For this review, take the finished solid that the model builds, in its own axes (mm). A direction names the side the tool comes from. Round coordinates to 2 decimals unless told otherwise and drop trailing zeros. Write each loop counter-clockwise with the first axis right and the second up, starting at its lowest first coordinate (ties: lowest second). Pieces come first, ordered by that corner, then holes.
from build123d import *

# Parameters (mm, degrees)
F0_R            = 10
F1_DEPTH        = 4
F3_DEPTH        = 4.001
F3_COPIES_COUNT = 9


# Not quite as in the source:
# - a pattern or mirror of a feature is missing from the dataset's text; its kind, count and spacing are read off the source's solid


with BuildPart() as f1:
    # F0 (on Top) → F1 (new body)
    with BuildSketch(Plane.XY):
        Circle(F0_R)
    extrude(amount=F1_DEPTH)

    # F2 (on face) → F3 (cut, through all)
    with BuildSketch(Plane.XY.offset(4)):
        with BuildLine():
            ThreePointArc((-2.7361611466, 7.5175409663), (-1.3891854213, 7.8784620241), (0, 8))
            Line((0, 8), (0, 10))
            ThreePointArc((0, 10), (-1.7364817767, 9.8480775301), (-3.4202014333, 9.3969262079))
            Line((-3.4202014333, 9.3969262079), (-2.7361611466, 7.5175409663))
        make_face()
    f3 = extrude(amount=-F3_DEPTH, mode=Mode.SUBTRACT)

    # F3_copies: F3 ×9 about axis
    f3_copies_axis = Axis((0, 0, 0), (0, 0, 1))
    for i in range(1, F3_COPIES_COUNT):
        add(f3.rotate(f3_copies_axis, i * 360 / F3_COPIES_COUNT), mode=Mode.SUBTRACT)


solid = f1.part
(1) We need section B-B, the plane x = 3. Give the boundary of the cut face in (y, z), and give its area (3 significant figures).
Geometry check:
outline: (-9.54, 0) - (-8.24, 0) - (-8.24, 4) - (-9.54, 4) - close; (-7.42, 0) - (7.42, 0) - (7.42, 4) - (-7.42, 4) - close; (8.24, 0) - (9.54, 0) - (9.54, 4) - (8.24, 4) - close
area: 69.7 mm2
(2) Mouldability with a two-part tool opening along X and no side actions: class faces 1 (the face through (8.877, -1.565, 2.028)), 2 (the face through (8, -6, 2)), 3 (the face through (-8.85, 1.56, 2.03)) as pulls with the +X half, pulls with the -X half, needs draft (parallel to the pull), parting line crosses it, or undercut.
Geometry check:
face 1: undercut
face 2: pulls with the +X half
face 3: pulls with the -X half
(3) We need section D-D, the plane x = -7.5. Give the boundary of the cut face in (y, z).
Geometry check:
outline: (-4.33, 0) - (4.33, 0) - (4.33, 4) - (-4.33, 4) - close
(4) We need section C-C, the plane y = 2.25. Give the boundary of the cut face in (x, z), and give its area (3 significant figures).
Geometry check:
outline: (-9.74, 0) - (7.68, 0) - (7.68, 4) - (-9.74, 4) - close
area: 69.7 mm2
(5) For faces 4 (the face through (-3.083, 8.47, 2.028)), 5 (the face through (-1.37, -7.88, 2.03)), 6 (the face through (-5.776, 6.884, 2.028)), list the 3-axis set-ups (+Z, -Z, +X, -X, +Y, -Y) from which the entire face can be reached by the end or side of a thin tool; tool diameter is ignored.
Geometry check:
face 4: +Z, -Z, +Y
face 5: +Z, -Z, -Y
face 6: +Z, -Z, -X
(6) We need section A-A, the plane y = -7. Give the boundary of the cut face in (x, z), and give its area (3 significant figures).
Geometry check:
outline: (-5.87, 0) - (3.87, 0) - (3.87, 4) - (-5.87, 4) - close; (5.87, 0) - (7.14, 0) - (7.14, 4) - (5.87, 4) - close
area: 44.1 mm2
(7) For line 1 along Y through (x, z) = (7.25, 1.55); line 2 along Y through (x, z) = (7, 0.7); line 3 along X through (y, z) = (4.75, 2), list the stretches that pass through material, from the lowest coordinate up.
Geometry check:
line 1: y = -6.89 to -4.19, -3.38 to 3.38, 4.19 to 6.89
line 2: y = -7.14 to -4.04, -3.87 to 3.87, 4.04 to 7.14
line 3: x = -8.8 to -8.23, -6.44 to 8.23
(8) For pin 1 Ø1 at (y, z) = (-2.5, 3) entering from +X; pin 2 Ø0.6 at (y, z) = (-8.5, 1.5) entering from -X; pin 3 Ø2 at (y, z) = (2, 3) entering from +X, all flat-tipped, find the tip position at first contact; note any pin that passes through.
Geometry check:
pin 1: stops at x = 7.75
pin 2: stops at x = -5.72
pin 3: stops at x = 9.95
